from build123d import *

# Parameters (mm, degrees)
SKETCH1_R           = 1.04
BOSS_EXTRUDE1_DEPTH = 6.5
SKETCH2_R           = 1.5
BOSS_EXTRUDE2_DEPTH = 2
CUT_EXTRUDE1_DEPTH  = 1.25
CHAMFER1_SIZE       = 0.25


with BuildPart() as part:
    # Sketch1 → Boss-Extrude1 (new body)
    with BuildSketch(Plane(origin=(0, 0, 0), x_dir=(1, 0, 0), z_dir=(0, 1, 0))):
        with Locations(Location((0, 0, 0), (0, 0, 90))):
            Circle(SKETCH1_R)
    extrude(amount=BOSS_EXTRUDE1_DEPTH)

    # Sketch2 → Boss-Extrude2 (add)
    with BuildSketch(Plane(origin=(0, 6.5, 0), x_dir=(1, 0, 0), z_dir=(0, 1, 0))):
        with Locations(Location((0, 0, 0), (0, 0, 270))):
            Circle(SKETCH2_R)
    extrude(amount=BOSS_EXTRUDE2_DEPTH)

    # Sketch3 → Cut-Extrude1 (cut)
    with BuildSketch(Plane(origin=(0, 8.5, 0), x_dir=(1, 0, 0), z_dir=(0, 1, 0))):
        Polygon((-0.032777471, 1.154235232), (-1.015985768, 0.548731493), (-0.983208297, -0.605503739), (0.032777471, -1.154235232), (1.015985768, -0.548731493), (0.983208297, 0.605503739), align=None)
    extrude(amount=-CUT_EXTRUDE1_DEPTH, mode=Mode.SUBTRACT)

    # Chamfer1
    chamfer1_edges = [part.edges().sort_by_distance(p)[0] for p in [
        (0, 0, 1.04),
    ]]
    chamfer(chamfer1_edges, length=CHAMFER1_SIZE)


solid = part.part
Geometry check sheet. Reference: the model listing, model coordinates, mm. A direction names the side the tool comes from. Give positions to 0.01 mm unless a question says otherwise; leave off trailing zeros. Write each loop counter-clockwise with the first axis right and the second up, starting at its lowest first coordinate (ties: lowest second). Pieces come first, ordered by that corner, then holes. Notation, with made-up numbers: M 69,50.25 L 74,50.25 A22 ccw 74,65.25 Z; hole C 26.25,46.25 d5. An arc over 180 degrees is marked long. Answer as CSV lines item,"result". Start each with the question number.
Q1. Material ranges on L1, parallel to Y at x = -0.15, z = 1.3; L2, parallel to Y at x = -0.1, z = -0.65; L3, parallel to X at y = 5.25, z = -0.05, recorded low to high.
Q2. Section check D-D, the plane x = 1.25. Record the cut outline in (y, z), then the cut area to 3 significant figures.
Q3. Tool access check on faces 1 (the face through (0.517, 7.884, 0.856)), 2 (the face through (0.45, 7.49, 1.43)). Record the directions out of +Z, -Z, +X, -X, +Y, -Y that give a thin tool (end or side, any length) a straight path to the whole face; none if there is none.
Q4. Section check A-A, the plane y = 8. Record the cut outline in (x, z), then the cut area to 3 significant figures.
Q5. Section check C-C, the plane y = 5. Record the cut outline in (x, z).
Q6. Section check B-B, the plane z = 0. Record the cut outline in (x, y).
Q7. Go/stop test with a flat-tipped pin: pin 1 (1 mm diameter, centred on x = 0, z = 0.5, fed in from +Y). Record where the tip stops, or that it passes through.
Q8. Release check for a two-part mould opening along Z. For faces 3 (the face through (0, 0, 0)), 4 (the face through (-0.482, 7.884, 0.876)), 5 (the face through (0.633, 3.331, 0.825)) record: pulls with the +Z half, pulls with the -Z half, needs draft (parallel to the pull), parting line crosses it, or undercut.
Geometry says:
1,L1,"6.5 to 8.5"
1,L2,"0 to 7.25"
1,L3,"-1.04 to 1.04"
2,outline,"M 6.5,-0.83 L 8.5,-0.83 L 8.5,0.83 L 6.5,0.83 Z"
2,area,"3.32 mm^2"
3,face 1,"+Y"
3,face 2,"+Y, -Y"
4,outline,"C 0,0 d3; hole M -1.02,-0.55 L -0.03,-1.15 L 0.98,-0.61 L 1.02,0.55 L 0.03,1.15 L -0.98,0.61 Z"
4,area,"3.60 mm^2"
5,outline,"C 0,0 d2.08"
6,outline,"M -1.5,6.5 L -1.04,6.5 L -1.04,0.25 L -0.79,0 L 0.79,0 L 1.04,0.25 L 1.04,6.5 L 1.5,6.5 L 1.5,8.5 L 1,8.5 L 1,7.25 L -1,7.25 L -1,8.5 L -1.5,8.5 Z"
7,pin 1,"y = 7.25"
8,face 3,"needs draft"
8,face 4,"undercut"
8,face 5,"parting line crosses it"
